from build123d import *

# Parameters (mm, degrees)
SKETCH1_R           = 6.35
BOSS_EXTRUDE1_DEPTH = 43.258347316


with BuildPart() as part:
    # Sketch1 → Boss-Extrude1 (new, symmetric)
    with BuildSketch(Plane.XY):
        Circle(SKETCH1_R)
    extrude(amount=BOSS_EXTRUDE1_DEPTH, both=True)

    # Sketch3 → Tap Drill for 1/4-20 Tap1 (revolve, cut)
    with BuildSketch(Plane(origin=(0, 0, 43.258347316), x_dir=(0, -1, 0), z_dir=(1, 0, 0))):
        Polygon((0, 0), (0, 17.408816902), (2.5527, 15.875), (2.5527, 0), align=None)
    tap_drill_for_1_4_20_tap1 = revolve(axis=Axis((0, 0, 49.608347316), (0, 0, -1)), mode=Mode.SUBTRACT)

    # Mirror1: Tap Drill for 1/4-20 Tap1 across plane
    add(tap_drill_for_1_4_20_tap1.mirror(Plane.XY), mode=Mode.SUBTRACT)


solid = part.part
Geometry check sheet. Reference: the model listing, model coordinates, mm. A direction names the side the tool comes from. Give positions to 0.01 mm unless a question says otherwise; leave off trailing zeros. Write each loop counter-clockwise with the first axis right and the second up, starting at its lowest first coordinate (ties: lowest second). Pieces come first, ordered by that corner, then holes. Notation, with made-up numbers: M 40.25,-19.5 L 52.25,-19.5 A28 ccw 52.25,13.5 Z; hole C -19.5,59 d2. An arc over 180 degrees is marked long. One line per question, with ' | ' between items.
1. Cross-section at D-D (y = -4.25). Enter the section's corners in (x, z).
Ans:
outline: M -4.72,-43.26 L 4.72,-43.26 L 4.72,43.26 L -4.72,43.26 Z
2. Scan lines: line 1 along Y through (x, z) = (0, -39); line 2 along X through (y, z) = (1, 37); line 3 along Y through (x, z) = (-0.75, 39.5). Record each from-to range of solid material in increasing order. Write a range as from..to.
Ans:
line 1: -6.35..-2.55, 2.55..6.35 | line 2: -6.27..-2.35, 2.35..6.27 | line 3: -6.31..-2.44, 2.44..6.31
3. Set-up check for faces 1 (the face through (-0.767, -2.435, -35.432)), 2 (the face through (-0.767, -2.435, 35.432)), 3 (the face through (3, 0, 43.258)): record each of +Z, -Z, +X, -X, +Y, -Y from which the full face is reachable in a straight line by a thin tool's end or side.
Ans:
face 1: -Z | face 2: +Z | face 3: +Z, +X, -X, +Y, -Y
4. Cross-section at B-B (x = -4.75). Enter the section's corners in (y, z).
Ans:
outline: M -4.21,-43.26 L 4.21,-43.26 L 4.21,43.26 L -4.21,43.26 Z
5. Cross-section at A-A (z = 34.5). Enter the section's corners in (x, y), plus the area to 3 significant figures.
Ans:
outline: C 0,0 d12.7; hole C 0,0 d5.11 | area: 106 mm2
6. Cross-section at C-C (z = 19.5). Enter the section's corners in (x, y), plus the area to 3 significant figures.
Ans:
outline: C 0,0 d12.7 | area: 127 mm2
7. Gauge pin test, flat ends, axial feed: pin 1 (4 mm diameter, centred on x = 4.5, z = -8, fed in from +Y); pin 2 (3 mm diameter, centred on x = 0, y = 0, fed in from -Z); pin 3 (1 mm diameter, centred on y = 1, z = -4.5, fed in from -X). Record the tip position at first contact, or that the pin passes through.
Ans:
pin 1: y = 5.84 | pin 2: z = -26.75 | pin 3: x = -6.33
8. Mould release check, pull along X, two halves, no side actions. Record for faces 4 (the face through (-1.38, -6.2, 0.61)), 5 (the face through (3, 0, -43.258)), 6 (the face through (-0.133, -0.423, -26.116)): released by +X, released by -X, zero draft, split by the parting line, or undercut.
Ans:
face 4: split by the parting line | face 5: zero draft | face 6: undercut
